Read the model definition and answer for the solid it produces. Units are mm, in the model's axes. Face numbers are marked on the shaded views. A direction names the side the tool comes from. Give positions to 0.01 mm unless a question says otherwise; leave off trailing zeros. Order: outer loops, then holes, each group sorted by start corner. A loop starts at its lowest first (then second) coordinate and runs counter-clockwise, first axis right, second up. Notation, with made-up numbers: (82, -7) -> (91, -7) arc R35 ccw to (91, 30) -> close; hole circle Ø9 at (52, 19). An arc over 180 degrees is marked (long way). One line per item, written item: value. Start each with the question number.
from build123d import *


with BuildPart() as part:
    # Esquisse1 → Révolution1 (revolve)
    with BuildSketch(Plane(origin=(0, 0, 0), x_dir=(0, 0, -1), z_dir=(1, 0, 0)), mode=Mode.PRIVATE) as r_volution1_sk:
        with BuildLine():
            Line((0, 2.25), (0.5, 2.25))
            Line((0.5, 2.25), (0.5, 4.65))
            Line((0.5, 4.65), (0.9, 4.65))
            Line((0.9, 4.65), (0.9, 12.35))
            Line((0.9, 12.35), (-2.1, 12.35))
            Line((-2.1, 12.35), (-2.2, 12.35))
            ThreePointArc((-2.2, 12.35), (-4.038477631, 11.588477631), (-4.8, 9.75))
            Line((-4.8, 9.75), (-4.8, 5.65))
            ThreePointArc((-4.8, 5.65), (-4.507106781, 4.942893219), (-3.8, 4.65))
            Line((-3.8, 4.65), (0, 4.65))
            Line((0, 4.65), (0, 2.25))
        make_face()
    revolve(r_volution1_sk.sketch.rotate(Axis((0, 0, 13.052048193), (0, 0, -1)), 90), axis=Axis((0, 0, 13.052048193), (0, 0, -1)))


solid = part.part
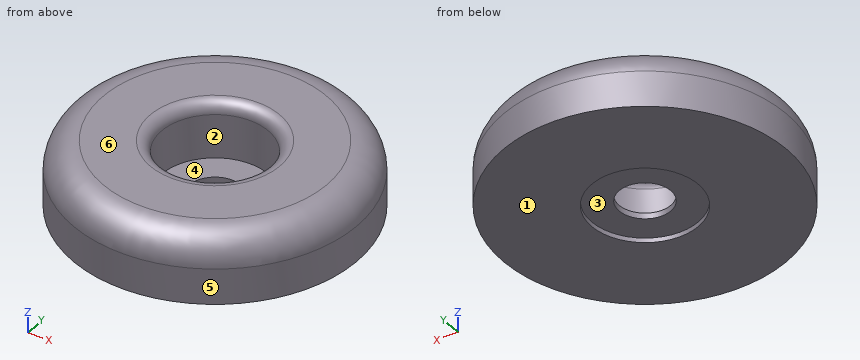
Item 1: Flat-ended cylindrical pins translate along their axes: pin 1 (6 mm diameter, centred on x = 0, y = 0, fed in from +Z); pin 2 (7.5 mm diameter, centred on x = 2, y = 2, fed in from +Z); pin 3 (1.5 mm diameter, centred on y = 9, z = 3.5, fed in from -X); pin 4 (8.5 mm diameter, centred on x = 0, y = 0, fed in from -Z). Find the tip coordinate at first contact, or state that the pin passes through.
Item 2: Find section C-C on z = 0.75. Write down the section's boundary in (x, y), then the cut area to 3 significant figures.
Item 3: A tool of negligible diameter and unlimited length cuts with its end or side. For the marked faces 1, 2 and 3, from which of +Z, -Z, +X, -X, +Y, -Y can it reach the whole face along a straight path? Write none if from no direction.
Item 4: Find section A-A on x = 0. Write down the section's boundary in (y, z).
Item 5: Find the intervals of material crossed by line 1 (Y direction, x = 0, z = -0.6); line 2 (Y direction, x = 0, z = -0.25); line 3 (X direction, y = -2.5, z = 1.9), in increasing order. Write a range as from..to.
Item 6: For a pull along Y with two mould halves and no side action, classify the marked faces 4, 5 and 6 as +Y half, -Y half, draft (parallel to the pull), parting line (faces both ways), or undercut.
Checks:
1. pin 1: z = 0
1. pin 2: z = 4.8
1. pin 3: x = -8.87
1. pin 4: z = -0.5
2. outline: circle Ø24.7 at (0, 0); hole circle Ø9.3 at (0, 0)
2. area: 411 mm2
3. face 1: -Z, +X, -X, +Y, -Y
3. face 2: +Z
3. face 3: -Z
4. outline: (-12.35, -0.9) -> (-4.65, -0.9) -> (-4.65, -0.5) -> (-2.25, -0.5) -> (-2.25, 0) -> (-4.65, 0) -> (-4.65, 3.8) arc R1 ccw to (-5.65, 4.8) -> (-9.75, 4.8) arc R2.6 ccw to (-12.35, 2.2) -> close; (2.25, -0.5) -> (4.65, -0.5) -> (4.65, -0.9) -> (12.35, -0.9) -> (12.35, 2.2) arc R2.6 ccw to (9.75, 4.8) -> (5.65, 4.8) arc R1 ccw to (4.65, 3.8) -> (4.65, 0) -> (2.25, 0) -> close
5. line 1: -12.35..-4.65, 4.65..12.35
5. line 2: -12.35..-2.25, 2.25..12.35
5. line 3: -12.09..-3.92, 3.92..12.09
6. face 4: undercut
6. face 5: parting line
6. face 6: draft
